```python
from build123d import *

# Parameters (mm, degrees)
CROQUIS1_R              = 4
SALIENTE_EXTRUIR1_DEPTH = 41
SALIENTE_EXTRUIR2_DEPTH = 6
CROQUIS3_R              = 3.9
SALIENTE_EXTRUIR3_DEPTH = 2.5
REDONDEO1_R             = 3


with BuildPart() as part:
    # Croquis1 → Saliente-Extruir1 (new body)
    with BuildSketch(Plane.XY):
        Circle(CROQUIS1_R)
    extrude(amount=SALIENTE_EXTRUIR1_DEPTH)

    # Croquis2 → Saliente-Extruir2 (add)
    with BuildSketch(Plane(origin=(0, 0, 0), x_dir=(-1, 0, 0), z_dir=(0, 0, -1))):
        Polygon((-2.309401077, 4), (-4.618802154, 0), (-2.309401077, -4), (2.309401077, -4), (4.618802154, 0), (2.309401077, 4), align=None)
    extrude(amount=SALIENTE_EXTRUIR2_DEPTH)

    # Croquis3 → Saliente-Extruir3 (add)
    with BuildSketch(Plane(origin=(0, 0, -6), x_dir=(-1, 0, 0), z_dir=(0, 0, -1))):
        Circle(CROQUIS3_R)
    extrude(amount=SALIENTE_EXTRUIR3_DEPTH)

    # Redondeo1
    redondeo1_edges = [part.edges().sort_by_distance(p)[0] for p in [
        (-4, 0, 41),
    ]]
    fillet(redondeo1_edges, radius=REDONDEO1_R)


solid = part.part
```
Part model, mm, in its own coordinate system. A direction names the side the tool comes from. Round coordinates to 2 decimals unless told otherwise and drop trailing zeros. Loops run counter-clockwise (first coordinate to the right, second up) from the corner with the lowest first, then second, coordinate; pieces in that order, holes last. Notation, with made-up numbers: (22.25, 74.5) -> (52.25, 74.5) arc R10 ccw to (52.25, 86.5) -> close; hole circle Ø3 at (-19.5, 36.25). An arc over 180 degrees is marked (long way). Use a Markdown table: item, result.
1) Drop flat-ended pins along their axis: pin 1 Ø1.6 at (x, y) = (2, 2.5) entering from +Z; pin 2 Ø5 at (x, z) = (3, 9.5) entering from +Y; pin 3 Ø1.6 at (x, y) = (1, -2.5) entering from +Z. Give the stop position or say it passes through.
The answers:
| item | result |
|---|---|
| pin 1 | stops at z = 40.65 |
| pin 2 | stops at y = 3.97 |
| pin 3 | stops at z = 40.86 |
2) Cut at A-A, the plane z = 10. List the corners of the cut face in (x, y).
The answers:
| item | result |
|---|---|
| outline | circle Ø8 at (0, 0) |
3) Tool access for faces 1 (the flat face through (2.1, 3.6, 0)), 2 (the flat face through (2.1, -3.6, 0)), 3 (the flat face through (-4.2, 0, 0)), 4 (the flat face through (-4.1, 0, -6)): list every direction of +Z, -Z, +X, -X, +Y, -Y with a clear straight run to the whole face (end or side of a thin tool).
The answers:
| item | result |
|---|---|
| face 1 | +Z, +X, +Y |
| face 2 | +Z, +X, -Y |
| face 3 | +Z, -X |
| face 4 | -Z |
4) Probe line 1 (X direction, y = -2, z = 5); line 2 (X direction, y = 0, z = 36); line 3 (Y direction, x = -2.5, z = 31). List the from-to ranges inside material, lowest first. Write a range as [from, to].
The answers:
| item | result |
|---|---|
| line 1 | x = [-3.46, 3.46] |
| line 2 | x = [-4, 4] |
| line 3 | y = [-3.12, 3.12] |
